from build123d import *

# Parameters (mm, degrees)
F0_W     = 20
F0_H     = 10
F0_W_2   = 30
F0_H_2   = 25
F1_DEPTH = 30
F2_START = -30
F2_DEPTH = 30


with BuildPart() as f1:
    # F0 (on Top) → F1 (new body)
    with BuildSketch(Plane.XY):
        with Locations((10, 5)):
            Rectangle(F0_W, F0_H)
        with Locations((10, 45)):
            Rectangle(F0_W, F0_H)
        Polygon((20, 10), (20, 0), (50, 0), (50, 25), (50, 50), (20, 50), (20, 40), align=None)
        with Locations((65, 37.5)):
            Rectangle(F0_W_2, F0_H_2)
    extrude(amount=-F1_DEPTH)

    # F0 (on Top) → F2 (join)
    with BuildSketch(Plane.XY.offset(F2_START)):
        Polygon((20, 10), (20, 0), (50, 0), (50, 25), (50, 50), (20, 50), (20, 40), align=None)
        with Locations((65, 37.5)):
            Rectangle(F0_W_2, F0_H_2)
        Polygon((80, 25), (80, 0), (110, 0), (110, 50), (80, 50), align=None)
        with Locations((65, 12.5)):
            Rectangle(F0_W_2, F0_H_2)
    extrude(amount=-F2_DEPTH)


solid = f1.part
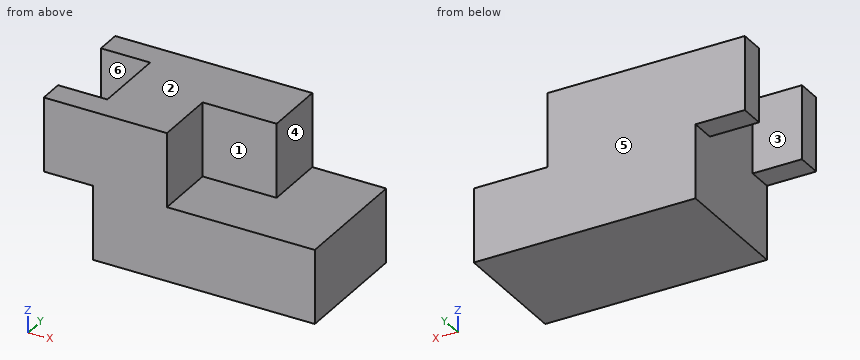
The model under review builds one solid part; all positions refer to its coordinate system, in mm. Face numbers are marked on the shaded views. A direction names the side the tool comes from. Round coordinates to 2 decimals unless told otherwise and drop trailing zeros. Write each loop counter-clockwise with the first axis right and the second up, starting at its lowest first coordinate (ties: lowest second). Pieces come first, ordered by that corner, then holes. Notation, with made-up numbers: (68, 71) - (121, 71) arc R37 cw to (121, 107) - close; hole circle Ø6 at (-21.75, -24). An arc over 180 degrees is marked (long way). One line per item, written item: value. Start each with the question number.
1. The part is to be moulded in two halves that separate along Y. For the marked faces 4, 5 and 6, say which applies: released by +Y, released by -Y, zero draft, split by the parting line, or undercut.
2. To check wall thickness, follow L1, parallel to Y at x = 13.5, z = -28; L2, parallel to X at y = 27, z = -27; L3, parallel to X at y = 15.5, z = -35.5. State the ranges of each line that lie inside material, in increasing order. Write a range as from..to.
3. Clearance check with flat-ended pins moving along their axes: P1, Ø3, axis at x = 39, y = 34, coming from the +Z side; P2, Ø7.5, axis at y = 38, z = -14, coming from the +X side; P3, Ø12.5, axis at y = 6.5, z = -13.5, coming from the +X side; P4, Ø3, axis at y = 35.5, z = -15, coming from the -X side. State where each tip first meets the part, or that it passes through.
4. Consider section B-B on z = -20. Write out the cut boundary in (x, y).
5. Machinability: for the marked faces 1, 2 and 3, which of the approach directions +Z, -Z, +X, -X, +Y, -Y give a long, thin tool a straight path to every point of the face, cutting with its end or side? Answer none if there is none.
6. Consider section D-D on x = 57. Write out the cut boundary in (y, z).
7. Consider section C-C on y = 22.5. Write out the cut boundary in (x, z).
8. Consider section A-A on x = 11. Write out the cut boundary in (y, z), and give its area (3 significant figures).
Checks:
1. face 4: zero draft
1. face 5: released by +Y
1. face 6: undercut
2. L1: y = 0..10, 40..50
2. L2: x = 20..80
2. L3: x = 20..110
3. P1: stops at z = 0
3. P2: stops at x = 80
3. P3: stops at x = 50
3. P4: stops at x = 20
4. outline: (0, 0) - (50, 0) - (50, 25) - (80, 25) - (80, 50) - (0, 50) - (0, 40) - (20, 40) - (20, 10) - (0, 10) - close
5. face 1: +Z, +X, -Y
5. face 2: +Z, +X, -X, +Y, -Y
5. face 3: +Z, -Z, -X
6. outline: (0, -60) - (50, -60) - (50, 0) - (25, 0) - (25, -30) - (0, -30) - close
7. outline: (20, -60) - (110, -60) - (110, -30) - (50, -30) - (50, 0) - (20, 0) - close
8. outline: (0, -30) - (10, -30) - (10, 0) - (0, 0) - close; (40, -30) - (50, -30) - (50, 0) - (40, 0) - close
8. area: 600 mm^2
